Could you check a few things on this model? Use its own coordinates, in mm. A direction names the side the tool comes from. Coordinates: 2 decimals unless noted, no trailing zeros. Loops run counter-clockwise (first coordinate to the right, second up) from the corner with the lowest first, then second, coordinate; pieces in that order, holes last. Notation, with made-up numbers: (59.25, 80.5) -> (99.25, 80.5) arc R25 cw to (99.25, 117.5) -> close; hole circle Ø11 at (41.5, 42). An arc over 180 degrees is marked (long way). One line per question, with ' | ' between items.
from build123d import *

# Parameters (mm, degrees)
F0_R     = 4.2
F1_DEPTH = 10
F5_D     = 8
F5_DEPTH = 15
F6_D     = 6.4
F6_DEPTH = 20
F7_SIZE  = 2


with BuildPart() as f1:
    # F0 (on Top) → F1 (new body)
    with BuildSketch(Plane.XY):
        Polygon((75, -129.903811), (150, 0), (75, 129.903811), (-75, 129.903811), (-150, 0), (-75, -129.903811), align=None)
        with Locations((-95.262794, -55)):
            Circle(F0_R, mode=Mode.SUBTRACT)
        with Locations((0, -110)):
            Circle(F0_R, mode=Mode.SUBTRACT)
        with Locations((95.262794, -55)):
            Circle(F0_R, mode=Mode.SUBTRACT)
        with Locations((-95.262794, 55)):
            Circle(F0_R, mode=Mode.SUBTRACT)
        with Locations((95.262794, 55)):
            Circle(F0_R, mode=Mode.SUBTRACT)
        with Locations((0, 110)):
            Circle(F0_R, mode=Mode.SUBTRACT)
    extrude(amount=F1_DEPTH)

    # F2 (on Front) → F3 (revolve, cut)
    with BuildSketch(Plane.XZ):
        Polygon((-23.5, 2), (-23.5, -10), (0, -10), (0, 18), (-60, 18), (-60, 8), (-22.5, 8), (-22.5, 6.5), (-13, 6.5), (-13, 2), align=None)
    revolve(axis=Axis((0, 0, -2.490325), (0, 0, -1)), mode=Mode.SUBTRACT)

    # F5
    with Locations(Plane.XY.offset(8)):
        with Locations((-26, 45.033321), (-52, 0), (-26, -45.033321), (26, -45.033321), (52, 0), (26, 45.033321), (-19.65, 34.034798), (-39.3, 0), (-19.65, -34.034798), (19.65, -34.034798), (39.3, 0), (19.65, 34.034798)):
            Hole(F5_D / 2, depth=F5_DEPTH)

    # F6
    with Locations(Plane.XY.offset(8)):
        with Locations((0, 52), (-45.033321, 26), (-45.033321, -26), (0, -52), (45.033321, -26), (45.033321, 26)):
            Hole(F6_D / 2, depth=F6_DEPTH)

    # F7
    f7_edges = [f1.edges().sort_by_distance(p)[0] for p in [
        (0, -129.903811, 10),
        (112.5, -64.951905, 10),
        (112.5, 64.951905, 10),
        (0, 129.903811, 10),
        (-112.5, 64.951905, 10),
        (-112.5, -64.951905, 10),
    ]]
    chamfer(f7_edges, length=F7_SIZE)


solid = f1.part
1) If we section it at D-D on x = -52: Please give me the cut outline in (y, z), and give its area (3 significant figures).
Data:
outline: (-129.9, 0) -> (-4, 0) -> (-4, 8) -> (-29.93, 8) -> (-29.93, 10) -> (-127.9, 10) -> (-129.9, 8) -> close; (4, 0) -> (129.9, 0) -> (129.9, 8) -> (127.9, 10) -> (29.93, 10) -> (29.93, 8) -> (4, 8) -> close | area: 2,410 mm²
2) We'd pull the mould along X, two halves only. Please class faces 1 (the face through (64, 2, 10)), 2 (the face through (-41.836, -25.859, 3.944)), 3 (the face through (112.15, 63.54, 9.01)): pulls with the +X half, pulls with the -X half, needs draft (parallel to the pull), parting line crosses it, or undercut.
Data:
face 1: needs draft | face 2: undercut | face 3: pulls with the +X half
3) I need wall thicknesses on line 1 along Y through (x, z) = (19.65, 2.25); line 2 along Y through (x, z) = (0, 3.7); line 3 along Y through (x, z) = (-39.3, 5). Which ranges of each line are inside material? Lowest first, please. Write a range as from..to.
Data:
line 1: -129.9..-38.03, -30.03..30.03, 38.03..129.9 | line 2: -129.9..-114.2, -105.8..-55.2, -48.8..-13, 13..48.8, 55.2..105.8, 114.2..129.9 | line 3: -129.9..-4, 4..129.9
4) If we section it at B-B on y = -17: Please give me the cut outline in (x, z), and give its area (3 significant figures).
Data:
outline: (-140.19, 0) -> (-16.22, 0) -> (-16.22, 2) -> (16.22, 2) -> (16.22, 0) -> (140.19, 0) -> (140.19, 8) -> (137.88, 10) -> (57.54, 10) -> (57.54, 8) -> (14.74, 8) -> (14.74, 6.5) -> (-14.74, 6.5) -> (-14.74, 8) -> (-57.54, 8) -> (-57.54, 10) -> (-137.88, 10) -> (-140.19, 8) -> close | area: 2,460 mm²
5) If we section it at C-C on x = -105.5: Please give me the cut outline in (y, z).
Data:
outline: (-77.08, 0) -> (77.08, 0) -> (77.08, 8) -> (73.08, 10) -> (-73.08, 10) -> (-77.08, 8) -> close
6) If we section it at A-A on x = 8: Please give me the cut outline in (y, z).
Data:
outline: (-129.9, 0) -> (-22.1, 0) -> (-22.1, 2) -> (-10.25, 2) -> (-10.25, 6.5) -> (-21.03, 6.5) -> (-21.03, 8) -> (-59.46, 8) -> (-59.46, 10) -> (-127.9, 10) -> (-129.9, 8) -> close; (10.25, 2) -> (22.1, 2) -> (22.1, 0) -> (129.9, 0) -> (129.9, 8) -> (127.9, 10) -> (59.46, 10) -> (59.46, 8) -> (21.03, 8) -> (21.03, 6.5) -> (10.25, 6.5) -> close
7) I'm going to push flat-ended pins straight in: pin 1 Ø3 at (y, z) = (75.5, 3) entering from -X; pin 2 Ø5 at (x, y) = (19.65, 34.03) entering from +Z; pin 3 Ø12 at (x, y) = (71, -18.5) entering from -Z; pin 4 Ø3 at (y, z) = (-82, 7.5) entering from +X. Where does each tip first touch, or does it pass through?
Data:
pin 1: x = -107.28 | pin 2: through | pin 3: z = 0 | pin 4: x = 103.52
8) On a 3-axis mill with a long thin cutter (end or side, diameter ignored), from which of +Z, -Z, +X, -X, +Y, -Y can I reach the whole of each face in a straight line? I mean faces 4 (the face through (10, -10, 2)), 5 (the face through (111.975, -65.861, 3.944)), 6 (the face through (59.94, 2.64, 8.99)). Say none if no direction works.
Data:
face 4: -Z | face 5: +Z, -Z, +X, -Y | face 6: +Z
